Read the model definition and answer for the solid it produces. Units are mm, in the model's axes. A direction names the side the tool comes from. Give positions to 0.01 mm unless a question says otherwise; leave off trailing zeros. Order: outer loops, then holes, each group sorted by start corner. A loop starts at its lowest first (then second) coordinate and runs counter-clockwise, first axis right, second up.
```python
from build123d import *

# Parameters (mm, degrees)
F0_W     = 200.152
F0_H     = 82.55
F1_DEPTH = 66.548
F3_DEPTH = 82.551
F5_DEPTH = 82.551
F7_DEPTH = 6.35
F8_DEPTH = 19.051
F9_R     = 3.175


with BuildPart() as f1:
    # F0 (on Top) → F1 (new body)
    with BuildSketch(Plane.XY):
        with Locations((33.701574, -19.847578)):
            Rectangle(F0_W, F0_H)
    extrude(amount=F1_DEPTH)

    # F2 (on face) → F3 (cut, through all)
    with BuildSketch(Plane.XZ.offset(61.122578)):
        Polygon((13.127574, 66.548), (-56.722426, 66.548), (-28.147426, 37.973), (-28.147426, 31.623), (-15.447426, 31.623), (-15.447426, 37.973), align=None)
    extrude(amount=-F3_DEPTH, mode=Mode.SUBTRACT)

    # F4 (on face) → F5 (cut, through all)
    with BuildSketch(Plane.XZ.offset(61.122578)):
        with BuildLine():
            Line((29.129574, 19.05), (133.777574, 19.05))
            Line((133.777574, 19.05), (133.777574, 66.548))
            Line((133.777574, 66.548), (22.779574, 66.548))
            Line((22.779574, 66.548), (22.779574, 25.4))
            ThreePointArc((22.779574, 25.4), (24.639446, 20.909872), (29.129574, 19.05))
        make_face()
    extrude(amount=-F5_DEPTH, mode=Mode.SUBTRACT)

    # F6 (on face) → F7 (join)
    with BuildSketch(Plane.XY.offset(19.05)):
        with BuildLine():
            Line((61.169598, -38.897577), (105.619598, -38.897577))
            ThreePointArc((105.619598, -38.897577), (124.669598, -19.847577), (105.619598, -0.797577))
            Line((105.619598, -0.797577), (61.169598, -0.797577))
            ThreePointArc((61.169598, -0.797577), (42.119598, -19.847577), (61.169598, -38.897577))
        make_face()
        with BuildLine():
            ThreePointArc((105.619598, -10.322577), (115.144598, -19.847577), (105.619598, -29.372577))
            Line((105.619598, -29.372577), (61.169598, -29.372577))
            ThreePointArc((61.169598, -29.372577), (51.644598, -19.847577), (61.169598, -10.322577))
            Line((61.169598, -10.322577), (105.619598, -10.322577))
        make_face(mode=Mode.SUBTRACT)
    extrude(amount=F7_DEPTH)

    # F7_face (on face) → F8 (cut, through all)
    with BuildSketch(Plane(origin=(83.394598, -19.847577, 19.05), x_dir=(1, 0, 0), z_dir=(0, 0, 1))):
        with BuildLine():
            ThreePointArc((-22.225, 9.525), (-31.75, 0), (-22.225, -9.525))
            Line((-22.225, -9.525), (22.225, -9.525))
            ThreePointArc((22.225, -9.525), (31.75, 0), (22.225, 9.525))
            Line((22.225, 9.525), (-22.225, 9.525))
        make_face()
    extrude(amount=-F8_DEPTH, mode=Mode.SUBTRACT)

    # F9
    f9_edges = [f1.edges().sort_by_distance(p)[0] for p in [
        (83.394598, -38.897577, 19.05),
        (42.119598, -19.847577, 19.05),
        (124.669598, -19.847577, 19.05),
        (83.394598, -10.322577, 25.4),
    ]]
    fillet(f9_edges, radius=F9_R)


solid = f1.part
```
1) The part is cut by section C-C on x = 91.5. Determine the outline of the cut face in (y, z) (3 decimals), and give its area (3 significant figures).
Final values:
outline: (-61.123, 0) - (-29.373, 0) - (-29.373, 22.225) arc R3.175 ccw to (-32.548, 25.4) - (-38.898, 25.4) - (-38.898, 22.225) arc R3.175 cw to (-42.073, 19.05) - (-61.123, 19.05) - close; (-10.323, 0) - (21.427, 0) - (21.427, 19.05) - (2.377, 19.05) arc R3.175 cw to (-0.798, 22.225) - (-0.798, 25.4) - (-7.148, 25.4) arc R3.175 ccw to (-10.323, 22.225) - close
area: 1,330 mm2
2) The part is cut by section A-A on z = 14.5. Determine the outline of the cut face in (x, y) (3 decimals).
Final values:
outline: (-66.374, -61.123) - (133.778, -61.123) - (133.778, 21.427) - (-66.374, 21.427) - close; hole (61.17, -29.373) - (105.62, -29.373) arc R9.525 ccw to (105.62, -10.323) - (61.17, -10.323) arc R9.525 ccw to start
3) For a pull along X with two mould halves and no side action, classify faces 1 (the face through (-42.635, -20.425, 52.461)), 2 (the face through (115.142, -20.057, 11.268)), 3 (the face through (133.778, -20, 9)), 4 (the face through (10, 21.427, 25)) as released by +X, released by -X, zero draft, split by the parting line, or undercut.
Final values:
face 1: undercut
face 2: undercut
face 3: released by +X
face 4: zero draft
4) The part is cut by section D-D on z = 43.5. Determine the outline of the cut face in (x, y).
Final values:
outline: (-66.37, -61.12) - (-33.67, -61.12) - (-33.67, 21.43) - (-66.37, 21.43) - close; (-9.92, -61.12) - (22.78, -61.12) - (22.78, 21.43) - (-9.92, 21.43) - close
5) Given pin 1 (6 mm diameter, centred on y = -24, z = 39, fed in from +X); pin 2 (1.6 mm diameter, centred on x = 75.5, z = 24, fed in from -Y); pin 3 (3.5 mm diameter, centred on x = 91, z = 23.5, fed in from +Y), each flat-ended and moving along its own axis, determine where each tip first touches the part or whether it passes through.
Final values:
pin 1: stops at x = 22.78
pin 2: stops at y = -38.9
pin 3: stops at y = -0.76
6) Consider L1, parallel to X at y = 8, z = 37.5; L2, parallel to Z at x = -23.5, y = -6; L3, parallel to Z at x = 120, y = -13.5. Determine where each line is inside the solid, lowest interval first.
Final values:
L1: x = -66.37 to -28.15, -15.45 to 22.78
L2: z = 0 to 31.62
L3: z = 0 to 25.4
7) A tool of negligible diameter and unlimited length cuts with its end or side. For faces 5 (the face through (42.124, -19.429, 23.79)), 6 (the face through (-1.36, -20.43, 52.06)), 7 (the face through (124.665, -20.266, 23.79)), from which of +Z, -Z, +X, -X, +Y, -Y can it reach the whole face along a straight path? Write none if from no direction.
Final values:
face 5: +Z
face 6: +Z, +Y, -Y
face 7: +Z, +X
8) The part is cut by section B-B on y = 14.5. Determine the outline of the cut face in (x, z), and give its area (3 significant figures).
Final values:
outline: (-66.37, 0) - (133.78, 0) - (133.78, 19.05) - (29.13, 19.05) arc R6.35 cw to (22.78, 25.4) - (22.78, 66.55) - (13.13, 66.55) - (-15.45, 37.97) - (-15.45, 31.62) - (-28.15, 31.62) - (-28.15, 37.97) - (-56.72, 66.55) - (-66.37, 66.55) - close
area: 6,800 mm2
